```python
from build123d import *

# Parameters (mm, degrees)
CROQUIS1_W              = 14
CROQUIS1_H              = 40
SALIENTE_EXTRUIR1_DEPTH = 9
CROQUIS3_R              = 2.675
CORTAR_EXTRUIR2_DEPTH   = 15
CROQUIS4_R              = 2.675
CORTAR_EXTRUIR3_DEPTH   = 15


with BuildPart() as part:
    # Croquis1 → Saliente-Extruir1 (new body)
    with BuildSketch(Plane(origin=(0, 0, 0), x_dir=(1, 0, 0), z_dir=(0, 1, 0))):
        Rectangle(CROQUIS1_W, CROQUIS1_H)
    extrude(amount=SALIENTE_EXTRUIR1_DEPTH)

    # Croquis3 → Cortar-Extruir2 (cut)
    with BuildSketch(Plane.XY.offset(20)):
        with Locations((-3.5, 4.5)):
            Circle(CROQUIS3_R)
        with Locations((3.5, 4.5)):
            Circle(CROQUIS3_R)
    extrude(amount=-CORTAR_EXTRUIR2_DEPTH, mode=Mode.SUBTRACT)

    # Croquis4 → Cortar-Extruir3 (cut, through all)
    with BuildSketch(Plane.ZY.offset(7)):
        with Locations((-15, 4.5)):
            Circle(CROQUIS4_R)
        with Locations((-6, 4.5)):
            Circle(CROQUIS4_R)
    extrude(amount=-CORTAR_EXTRUIR3_DEPTH, mode=Mode.SUBTRACT)


solid = part.part
```
The model under review builds one solid part; all positions refer to its coordinate system, in mm. A direction names the side the tool comes from. Round coordinates to 2 decimals unless told otherwise and drop trailing zeros. Loops run counter-clockwise (first coordinate to the right, second up) from the corner with the lowest first, then second, coordinate; pieces in that order, holes last. Notation, with made-up numbers: M -26,-24 L -1,-24 A20 cw -1,-13 Z; hole C 75,-8.75 d9. An arc over 180 degrees is marked long. Answer as a JSON object with one key per item and string values.
(1) Take a section at C-C on x = -3.5. Give the boundary of the cut face in (y, z) (3 decimals), and give its area (3 significant figures).
Resolved:
{"outline": "M 0,-20 L 9,-20 L 9,20 L 7.175,20 L 7.175,5 L 1.825,5 L 1.825,20 L 0,20 Z; hole C 4.5,-15 d5.35; hole C 4.5,-6 d5.35", "area": "235 mm²"}
(2) To check wall thickness, follow line 1 along Z through (x, y) = (1, 5.75); line 2 along Y through (x, z) = (-3.5, 14) (3 decimals); line 3 along Z through (x, y) = (-4.75, 6.75). State the ranges of each line that lie inside material, in increasing order.
Resolved:
{"line 1": "-20 to -17.36, -12.64 to -8.36, -3.64 to 20", "line 2": "0 to 1.825, 7.175 to 9", "line 3": "-20 to -16.45, -13.55 to -7.45, -4.55 to 5"}
(3) Take a section at D-D on z = 15. Give the boundary of the cut face in (x, y) (3 decimals), and give its area (3 significant figures).
Resolved:
{"outline": "M -7,0 L 7,0 L 7,9 L -7,9 Z; hole C -3.5,4.5 d5.35; hole C 3.5,4.5 d5.35", "area": "81.0 mm²"}
(4) Take a section at A-A on z = -6. Give the boundary of the cut face in (x, y) (3 decimals), and give its area (3 significant figures).
Resolved:
{"outline": "M -7,0 L 7,0 L 7,1.825 L -7,1.825 Z; M -7,7.175 L 7,7.175 L 7,9 L -7,9 Z", "area": "51.1 mm²"}
(5) Take a section at B-B on y = 4.5. Give the boundary of the cut face in (x, z) (3 decimals), and give its area (3 significant figures).
Resolved:
{"outline": "M -7,-20 L 7,-20 L 7,-17.675 L -7,-17.675 Z; M -7,-12.325 L 7,-12.325 L 7,-8.675 L -7,-8.675 Z; M -7,-3.325 L 7,-3.325 L 7,20 L 6.175,20 L 6.175,5 L 0.825,5 L 0.825,20 L -0.825,20 L -0.825,5 L -6.175,5 L -6.175,20 L -7,20 Z", "area": "250 mm²"}
(6) Tool access review of faces 1 (the flat face through (-7, 4, 0)), 2 (the cylindrical face through (-2.266, 2.127, 12.605)): name each direction out of +Z, -Z, +X, -X, +Y, -Y from which nothing blocks a thin tool from reaching the whole face with its end or side.
Resolved:
{"face 1": "+Z, -Z, -X, +Y, -Y", "face 2": "+Z"}
(7) Clearance check with flat-ended pins moving along their axes: P1, Ø4.5, axis at x = -3.5, y = 4.5, coming from the +Z side; P2, Ø3, axis at y = 4.5, z = -6, coming from the -X side. State where each tip first meets the part, or that it passes through.
Resolved:
{"P1": "z = 5", "P2": "through"}
(8) Draft analysis for pull direction X (two halves, no side actions). For faces 3 (the flat face through (0, 4, 20)), 4 (the cylindrical face through (1.38, 2.87, 12.6)), 5 (the flat face through (-4, 5, 5)), 6 (the flat face through (7, 4, 0)), state which applies: released by +X, released by -X, zero draft, split by the parting line, or undercut.
Resolved:
{"face 3": "zero draft", "face 4": "undercut", "face 5": "undercut", "face 6": "released by +X"}
